CAD build for the part. Positions are in the model's coordinates, mm. Face numbers are marked on the shaded views. A direction names the side the tool comes from. Give positions to 0.01 mm unless a question says otherwise; leave off trailing zeros. Write each loop counter-clockwise with the first axis right and the second up, starting at its lowest first coordinate (ties: lowest second). Pieces come first, ordered by that corner, then holes. Notation, with made-up numbers: (-3.75, 66) -> (10.25, 66) arc R23 ccw to (10.25, 96) -> close; hole circle Ø5 at (13.5, -25.5). An arc over 180 degrees is marked (long way). Answer as a JSON object with one key per item and string values.
```python
from build123d import *

# Parameters (mm, degrees)
F0_R           = 5
F1_DEPTH       = 82
F4_DEPTH       = 4
F6_R           = 5.5
F6_R_2         = 4.5
F7_DEPTH       = 11
F7_DEPTH_BACK  = 1
F9_R           = 5.5
F9_R_2         = 4.5
F10_DEPTH      = 11
F10_DEPTH_BACK = 1
F11_DEPTH      = 5
F13_R          = 7.5
F14_DEPTH      = 16.5
F14_DEPTH_BACK = 16.5
F16_DEPTH      = 1


with BuildPart() as f1:
    # F0 (on Front) → F1 (new body)
    with BuildSketch(Plane.XZ):
        Circle(F0_R)
    extrude(amount=F1_DEPTH)

    # F3 (on face) → F4 (join)
    with BuildSketch(Plane(origin=(0, 0, 0), x_dir=(-1, 0, 0), z_dir=(0, 1, 0))):
        Polygon((2.886751, 5), (-2.886751, 5), (-5.773503, 0), (-2.886751, -5), (2.886751, -5), (5.773503, 0), align=None)
    extrude(amount=-F4_DEPTH)

    # F6 (on offset) → F7 (cut, two sides)
    with BuildSketch(Plane.XZ.offset(13.5)) as f7_sk:
        Circle(F6_R)
        Circle(F6_R_2, mode=Mode.SUBTRACT)
    extrude(amount=F7_DEPTH, mode=Mode.SUBTRACT)
    extrude(f7_sk.sketch, amount=-F7_DEPTH_BACK, mode=Mode.SUBTRACT)

    # F9 (on offset) → F10 (cut, two sides)
    with BuildSketch(Plane.XZ.offset(58.5)) as f10_sk:
        Circle(F9_R)
        Circle(F9_R_2, mode=Mode.SUBTRACT)
    extrude(amount=F10_DEPTH, mode=Mode.SUBTRACT)
    extrude(f10_sk.sketch, amount=-F10_DEPTH_BACK, mode=Mode.SUBTRACT)

    # F2 (on face) → F11 (join)
    with BuildSketch(Plane.XZ.offset(82)):
        Polygon((2.886751, 5), (-2.886751, 5), (-5.773503, 0), (-2.886751, -5), (2.886751, -5), (5.773503, 0), align=None)
    extrude(amount=F11_DEPTH)

    # F13 (on offset) → F14 (join, two sides)
    with BuildSketch(Plane.XZ.offset(41)) as f14_sk:
        Circle(F13_R)
    extrude(amount=F14_DEPTH)
    extrude(f14_sk.sketch, amount=-F14_DEPTH_BACK)

    # F15 (on face) → F16 (join)
    with BuildSketch(Plane(origin=(0, 0, 0), x_dir=(-1, 0, 0), z_dir=(0, 1, 0))):
        Polygon((5.773503, 0), (2.886751, 5), (-2.886751, 5), (-5.773503, 0), (-2.886751, -5), (2.886751, -5), align=None)
    extrude(amount=F16_DEPTH)


solid = f1.part
```
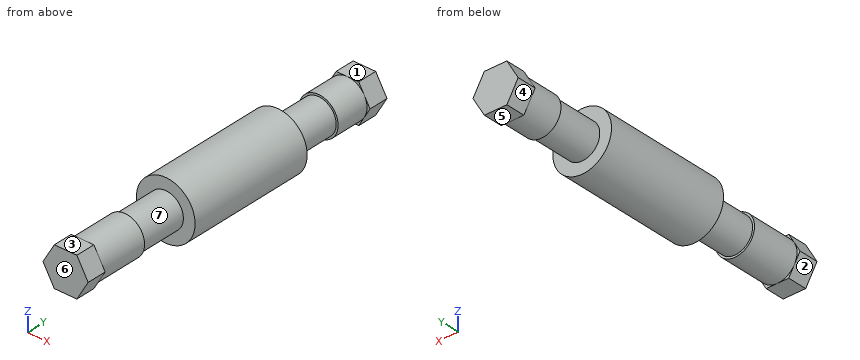
1) Slice it at B-B (z = 6). List the corners of the cut face in (x, y).
Model answer:
{"outline": "(-4.5, -57.5) -> (4.5, -57.5) -> (4.5, -24.5) -> (-4.5, -24.5) -> close"}
2) Slice it at C-C (y = -55). List the corners of the cut face in (x, z), then the cut area to 3 significant figures.
Model answer:
{"outline": "circle Ø15 at (0, 0)", "area": "177 mm2"}
3) Pin check, flat tips, straight feed: pin 1 (4 mm diameter, centred on x = -1, y = -1.5, fed in from -Z); pin 2 (5 mm diameter, centred on y = -23.5, z = 3, fed in from -X); pin 3 (1.5 mm diameter, centred on x = 0.5, y = -83.5, fed in from +Z). Stop position of each tip, or through.
Model answer:
{"pin 1": "stops at z = -5", "pin 2": "stops at x = -7.47", "pin 3": "stops at z = 5"}
4) 3-axis set-ups, long thin cutter, end or side, ignore diameter. For the marked faces 1, 2, 3 and 4: which of +Z, -Z, +X, -X, +Y, -Y reach the whole face in a straight line?
Model answer:
{"face 1": "+Z, +X, -X, +Y", "face 2": "-Z, -X, -Y", "face 3": "+Z, +X, -X, -Y", "face 4": "-Z, -X, +Y"}
5) Wall check: probe 1 along Y at (x, z) = (3, 5.5); probe 2 along X at (y, z) = (-50.5, -0.5); probe 3 along Z at (x, y) = (-4, -78). Give the ranges that are in metal, low to high.
Model answer:
{"probe 1": "y = -57.5 to -24.5", "probe 2": "x = -7.48 to 7.48", "probe 3": "z = -3 to 3"}
6) Mould opens along Y. For the marked faces 5, 6 and 7 say: released by +Y, released by -Y, zero draft, split by the parting line, or undercut.
Model answer:
{"face 5": "zero draft", "face 6": "released by -Y", "face 7": "undercut"}
7) Slice it at A-A (x = 1.25). List the corners of the cut face in (y, z).
Model answer:
{"outline": "(-87, -5) -> (-82, -5) -> (-82, -4.84) -> (-69.5, -4.84) -> (-69.5, -4.32) -> (-57.5, -4.32) -> (-57.5, -7.4) -> (-24.5, -7.4) -> (-24.5, -4.32) -> (-12.5, -4.32) -> (-12.5, -4.84) -> (-4, -4.84) -> (-4, -5) -> (1, -5) -> (1, 5) -> (-4, 5) -> (-4, 4.84) -> (-12.5, 4.84) -> (-12.5, 4.32) -> (-24.5, 4.32) -> (-24.5, 7.4) -> (-57.5, 7.4) -> (-57.5, 4.32) -> (-69.5, 4.32) -> (-69.5, 4.84) -> (-82, 4.84) -> (-82, 5) -> (-87, 5) -> close"}
8) Slice it at D-D (y = -8.5). List the corners of the cut face in (x, z).
Model answer:
{"outline": "circle Ø10 at (0, 0)"}
